Read the model definition and answer for the solid it produces. Units are mm, in the model's axes. A direction names the side the tool comes from. Coordinates: 2 decimals unless noted, no trailing zeros. Loops run counter-clockwise (first coordinate to the right, second up) from the corner with the lowest first, then second, coordinate; pieces in that order, holes last. Notation, with made-up numbers: M 57.5,-20 L 78.5,-20 A17 ccw 78.5,0 Z; hole C -29.75,78 d8. An arc over 180 degrees is marked long. One line per item, written item: value. Start each with the question number.
1. Consider probe 1 along Y at (x, z) = (66.15, 1.1); probe 2 along X at (y, z) = (-20.5, 10.5); probe 3 along Z at (x, y) = (89, -42). Determine where each line is inside the solid, lowest interval first.
2. The part is cut by section A-A (x = 71.5). Write down the section's boundary in (y, z).
3. The part is cut by section C-C (y = -24). Write down the section's boundary in (x, z), then the cut area to 3 significant figures.
4. Flat-ended cylindrical pins translate along their axes: pin 1 (3.5 mm diameter, centred on x = -2, y = -51, fed in from -Z); pin 2 (0.6 mm diameter, centred on y = -50.5, z = -1, fed in from +X); pin 3 (6 mm diameter, centred on x = 30.5, y = -6.5, fed in from -Z). Find the tip coordinate at first contact, or state that the pin passes through.
5. For faces 4 (the face through (17.5, -21, 21)), 5 (the face through (14.7, -45, -1)), 6 (the face through (-2, -15, 3.2)), 7 (the face through (3.7, -45, -1)), determine the directions among +Z, -Z, +X, -X, +Y, -Y from which every point of the face is accessible in a straight line to the end or side of a thin tool.
6. The part is cut by section B-B (z = 21.5). Write down the section's boundary in (x, y).
7. Determine the mould class of faces 1 (the face through (-2, -19.4, 6)), 2 (the face through (92.174, -3.182, 15.538)), 3 (the face through (50, -26, 0)) for opening direction Z: +Z half, -Z half, draft (parallel to the pull), parting line (faces both ways), or undercut.
```python
from build123d import *

# Parameters (mm, degrees)
F0_R      = 1.65
F1_DEPTH  = 1.7
F3_DEPTH  = 2.3
F4_W      = 66.6
F4_H      = 2.7
F4_W_2    = 70.5
F4_W_3    = 5
F4_H_2    = 46.2
F5_DEPTH  = 13
F4_W_4    = 10.3
F4_H_3    = 12
F4_W_5    = 6
F6_DEPTH  = 11
F4_W_6    = 13
F4_H_4    = 8
F4_W_7    = 1
F7_DEPTH  = 11
F8_W      = 9
F8_H      = 8
F9_DEPTH  = 7.9
F10_R     = 3.1
F10_R_2   = 0.5
F11_DEPTH = 4.5
F12_SIZE  = 3
F13_W     = 6
F13_H     = 3
F14_DEPTH = 7.9
F16_W     = 101.7
F16_H     = 60.5
F16_R     = 1.65
F17_DEPTH = 1.7
F18_W     = 7.5
F18_H     = 30
F19_DEPTH = 9
F18_W_2   = 9
F18_H_2   = 20.5
F18_W_3   = 3
F20_DEPTH = 8


with BuildPart() as f1:
    # F0 (on Top) → F1 (new body)
    with BuildSketch(Plane.XY):
        Polygon((96.4, 0), (0, 0), (0, -8.9), (0, -20.9), (0, -40.5), (0, -49.5), (0, -53.5), (98.9, -53.5), (98.9, -52.5), (101.5, -49.9), (101.5, -15.1), (98.9, -12.5), (98.9, -2.5), align=None)
        with Locations((14.35, -50.85)):
            Circle(F0_R, mode=Mode.SUBTRACT)
        with Locations((66.15, -45.75)):
            Circle(F0_R, mode=Mode.SUBTRACT)
        with Locations((96.8263558647, -50.85)):
            Circle(F0_R, mode=Mode.SUBTRACT)
        with Locations((15.75, -2.55)):
            Circle(F0_R, mode=Mode.SUBTRACT)
        with Locations((66.15, -17.75)):
            Circle(F0_R, mode=Mode.SUBTRACT)
        with Locations((90.65, -2.55)):
            Circle(F0_R, mode=Mode.SUBTRACT)
    extrude(amount=F1_DEPTH)

    # F2 (on face) → F3 (join)
    with BuildSketch(Plane(origin=(0, 0, 0), x_dir=(1, 0, 0), z_dir=(0, 0, -1))):
        Polygon((10.2355339059, 52.5), (8.1644660941, 52.5), (6.7, 51.0355339059), (6.7, 48.9644660941), (8.1644660941, 47.5), (10.2355339059, 47.5), (11.7, 48.9644660941), (11.7, 51.0355339059), align=None)
        Polygon((7.2355339059, 47.0147186258), (5.1644660941, 47.0147186258), (3.7, 45.5502525317), (3.7, 43.4791847198), (5.1644660941, 42.0147186258), (7.2355339059, 42.0147186258), (8.7, 43.4791847198), (8.7, 45.5502525317), align=None)
        Polygon((13.2355339059, 47.0147186258), (11.1644660941, 47.0147186258), (9.7, 45.5502525317), (9.7, 43.4791847198), (11.1644660941, 42.0147186258), (13.2355339059, 42.0147186258), (14.7, 43.4791847198), (14.7, 45.5502525317), align=None)
    extrude(amount=F3_DEPTH)

    # F4 (on face) → F5 (join)
    with BuildSketch(Plane.XY.offset(1.7)):
        with Locations((55.1, -51.65)):
            Rectangle(F4_W, F4_H)
        with Locations((53.65, -1.85)):
            Rectangle(F4_W_2, F4_H)
        with Locations((95.15, -24.35)):
            Rectangle(F4_W_3, F4_H_2)
    extrude(amount=F5_DEPTH)

    # F4 (on face) → F6 (join)
    with BuildSketch(Plane.XY.offset(1.7)):
        with Locations((5.15, -14.9)):
            Rectangle(F4_W_4, F4_H_3)
        with Locations((-3, -14.9)):
            Rectangle(F4_W_5, F4_H_3)
    extrude(amount=F6_DEPTH)

    # F4 (on face) → F7 (join)
    with BuildSketch(Plane.XY.offset(1.7)):
        with Locations((6.5, -45.5)):
            Rectangle(F4_W_6, F4_H_4)
        with Locations((-0.5, -45.5)):
            Rectangle(F4_W_7, F4_H_4)
    extrude(amount=F7_DEPTH)

    # F8 (on face) → F9 (cut)
    with BuildSketch(Plane(origin=(-6, 0, 0), x_dir=(0, -1, 0), z_dir=(-1, 0, 0))):
        with Locations((14.9, 7.2)):
            Rectangle(F8_W, F8_H)
    extrude(amount=-F9_DEPTH, mode=Mode.SUBTRACT)

    # F10 (on face) → F11 (cut)
    with BuildSketch(Plane(origin=(-1, 0, 0), x_dir=(0, -1, 0), z_dir=(-1, 0, 0))):
        with Locations((45.5, 8.7)):
            Circle(F10_R)
        with Locations((45.5, 8.7)):
            Circle(F10_R_2, mode=Mode.SUBTRACT)
    extrude(amount=-F11_DEPTH, mode=Mode.SUBTRACT)

    # F12
    f12_edges = [f1.edges().sort_by_distance(p)[0] for p in [
        (-2.05, -10.4, 11.2),
        (-2.05, -19.4, 11.2),
    ]]
    chamfer(f12_edges, length=F12_SIZE)

    # F13 (on face) → F14 (join, through all)
    with BuildSketch(Plane(origin=(1.9, 0, 0), x_dir=(0, -1, 0), z_dir=(-1, 0, 0))):
        with Locations((14.9, 7.4)):
            Rectangle(F13_W, F13_H)
    extrude(amount=F14_DEPTH)

    # F16 (on offset) → F17 (join)
    with BuildSketch(Plane.XY.offset(14.7)):
        with Locations((50.85, -30.25)):
            Rectangle(F16_W, F16_H)
        with Locations((14.35, -50.85)):
            Circle(F16_R, mode=Mode.SUBTRACT)
        with Locations((15.75, -2.55)):
            Circle(F16_R, mode=Mode.SUBTRACT)
        with Locations((90.65, -2.55)):
            Circle(F16_R, mode=Mode.SUBTRACT)
    extrude(amount=F17_DEPTH)

    # F18 (on face) → F19 (join)
    with BuildSketch(Plane.XY.offset(16.4)):
        with Locations((13.75, -21)):
            Rectangle(F18_W, F18_H)
    extrude(amount=F19_DEPTH)

    # F18 (on face) → F20 (join)
    with BuildSketch(Plane.XY.offset(16.4)):
        with Locations((4.5, -47.75)):
            Rectangle(F18_W_2, F18_H_2)
        with Locations((-1.5, -47.75)):
            Rectangle(F18_W_3, F18_H_2)
    extrude(amount=F20_DEPTH)


solid = f1.part
```
Answer block:
1. probe 1: y = -53.5 to -47.4, -44.1 to -19.4, -16.1 to 0
1. probe 2: x = -6 to 10.3, 92.65 to 97.65
1. probe 3: z = 0 to 1.7, 14.7 to 16.4
2. outline: M -60.5,14.7 L -53,14.7 L -53,1.7 L -53.5,1.7 L -53.5,0 L 0,0 L 0,1.7 L -0.5,1.7 L -0.5,14.7 L 0,14.7 L 0,16.4 L -60.5,16.4 Z; hole M -50.3,1.7 L -3.2,1.7 L -3.2,14.7 L -50.3,14.7 Z
3. outline: M 0,0 L 101.5,0 L 101.5,1.7 L 97.65,1.7 L 97.65,14.7 L 101.7,14.7 L 101.7,16.4 L 17.5,16.4 L 17.5,25.4 L 10,25.4 L 10,16.4 L 0,16.4 L 0,14.7 L 92.65,14.7 L 92.65,1.7 L 0,1.7 Z
3. area: 478 mm2
4. pin 1: stops at z = 16.4
4. pin 2: stops at x = 11.7
4. pin 3: stops at z = 0
5. face 4: +Z, +X, +Y, -Y
5. face 5: -Z, +X, +Y, -Y
5. face 6: -X
5. face 7: -Z, -X, +Y, -Y
6. outline: M -3,-58 L 9,-58 L 9,-37.5 L -3,-37.5 Z; M 10,-36 L 17.5,-36 L 17.5,-6 L 10,-6 Z
7. face 1: undercut
7. face 2: draft
7. face 3: -Z half
